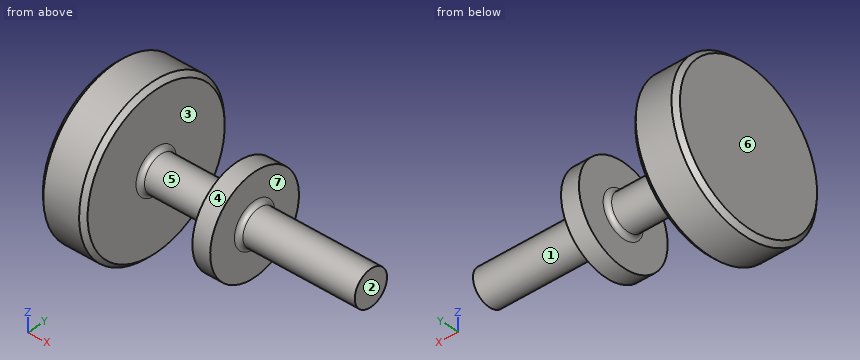
```python
from build123d import *

# Parameters (mm, degrees)
CHAMFER1_SIZE = 1
FILLET1_R     = 1


with BuildPart() as part:
    # Sketch1 → Revolve1 (revolve)
    with BuildSketch(Plane.XY, mode=Mode.PRIVATE) as revolve1_sk:
        Polygon((0, 0), (0, 18), (10, 18), (10, 4), (28, 4), (28, 11), (32, 11), (32, 4), (58, 4), (58, 0), align=None)
    revolve(revolve1_sk.sketch.rotate(Axis((0, 0, 0), (1, 0, 0)), 90), axis=Axis((0, 0, 0), (1, 0, 0)))

    # Chamfer1
    chamfer1_edges = [part.edges().sort_by_distance(p)[0] for p in [
        (10, 0, -18),
        (0, 0, -18),
    ]]
    chamfer(chamfer1_edges, length=CHAMFER1_SIZE)

    # Fillet1
    fillet1_edges = [part.edges().sort_by_distance(p)[0] for p in [
        (28, 0, -4),
        (10, 0, -4),
        (32, 0, -4),
    ]]
    fillet(fillet1_edges, radius=FILLET1_R)


solid = part.part
```
The listing builds one solid part. Answer for the finished solid, in the listing's coordinates (mm). Face numbers are marked on the shaded views. A direction names the side the tool comes from. Round coordinates to 2 decimals unless told otherwise and drop trailing zeros. Loops run counter-clockwise (first coordinate to the right, second up) from the corner with the lowest first, then second, coordinate; pieces in that order, holes last.
Q1. Given pin 1 Ø12 at (x, y) = (46, -3.5) entering from -Z; pin 2 Ø6 at (y, z) = (10.5, 12) entering from +X; pin 3 Ø1.5 at (x, z) = (21, 3) entering from -Y, each flat-ended and moving along its own axis, determine where each tip first touches the part or whether it passes through.
Q2. Section A-A, the plane y = 0 is taken. Determine the outline of the cut face in (x, z), then the cut area to 3 significant figures.
Q3. For a pull along X with two mould halves and no side action, classify the marked faces 4, 5, 6 and 7 as released by +X, released by -X, zero draft, split by the parting line, or undercut.
Q4. Which of the six approach directions +Z, -Z, +X, -X, +Y, -Y give full straight-line access (tool end or side, diameter ignored) to the marked faces 1, 2 and 3?
Q5. Find the intervals of material crossed by line 1 (X direction, y = -5, z = 7); line 2 (X direction, y = -15, z = 0.5); line 3 (X direction, y = 3, z = 3.5), in increasing order.
Q6. Section D-D, the plane x = 48.5 is taken. Determine the outline of the cut face in (y, z), then the cut area to 3 significant figures.
Q7. Section C-C, the plane x = 6 is taken. Determine the outline of the cut face in (y, z), then the cut area to 3 significant figures.
Completed:
1. pin 1: stops at z = -4
1. pin 2: stops at x = 10
1. pin 3: stops at y = -3.31
2. outline: (0, -17) - (1, -18) - (9, -18) - (10, -17) - (10, -5) arc R1 cw to (11, -4) - (27, -4) arc R1 cw to (28, -5) - (28, -11) - (32, -11) - (32, -5) arc R1 cw to (33, -4) - (58, -4) - (58, 4) - (33, 4) arc R1 cw to (32, 5) - (32, 11) - (28, 11) - (28, 5) arc R1 cw to (27, 4) - (11, 4) arc R1 cw to (10, 5) - (10, 17) - (9, 18) - (1, 18) - (0, 17) - close
2. area: 799 mm2
3. face 4: zero draft
3. face 5: undercut
3. face 6: released by -X
3. face 7: released by +X
4. face 1: +X
4. face 2: +Z, -Z, +X, +Y, -Y
4. face 3: none
5. line 1: x = 0 to 10, 28 to 32
5. line 2: x = 0 to 10
5. line 3: x = 0 to 10.08, 27.92 to 32.08
6. outline: circle Ø8 at (0, 0)
6. area: 50.3 mm2
7. outline: circle Ø36 at (0, 0)
7. area: 1,020 mm2
